Input: dimensioned drawing with shaded views. Units: mm. Origin: part minimum x, y, z. A direction names the side the tool comes from. Coordinates: 2 decimals unless noted, no trailing zeros. Loops run counter-clockwise (first coordinate to the right, second up) from the corner with the lowest first, then second, coordinate; pieces in that order, holes last.
Item 1: Section query B-B, the plane y = 17. Return the cut outline in (x, z), then the cut area to 3 significant figures.
Item 2: Reachability of the marked faces 1, 2, 3 and 4 from +Z, -Z, +X, -X, +Y, -Y: full face, straight path, thin tool, end or side. Return the list, or none.
Item 3: Pin query (flat end, axial travel): pin 1 Ø8 at (x, z) = (59.5, 18) entering from +Y; pin 2 Ø3 at (y, z) = (24, 15) entering from +X; pin 3 Ø5.5 at (y, z) = (8, 73.5) entering from -X; pin 4 Ø3 at (x, z) = (3.5, 75) entering from -Y. Return the tip coordinate at first contact, or that it passes through.
Item 4: Section query A-A, the plane x = 38.5. Return the cut outline in (y, z), then the cut area to 3 significant figures.
Item 5: Section query C-C, the plane x = 91. Return the cut outline in (y, z).
Item 6: Line query: probe 1 along Z at (x, y) = (34.5, 12); probe 2 along Z at (x, y) = (29, 21.25); probe 3 along Y at (x, z) = (63.5, 80). Output: solid intervals per line, ascending.
Item 7: Pull-direction query (X, two-part tool) for the marked faces 5, 6, 7 and 8; classes: +X half, -X half, draft (parallel to the pull), parting line (faces both ways), or undercut.
Item 8: Section query D-D, the plane z = 71. Return the cut outline in (x, y).
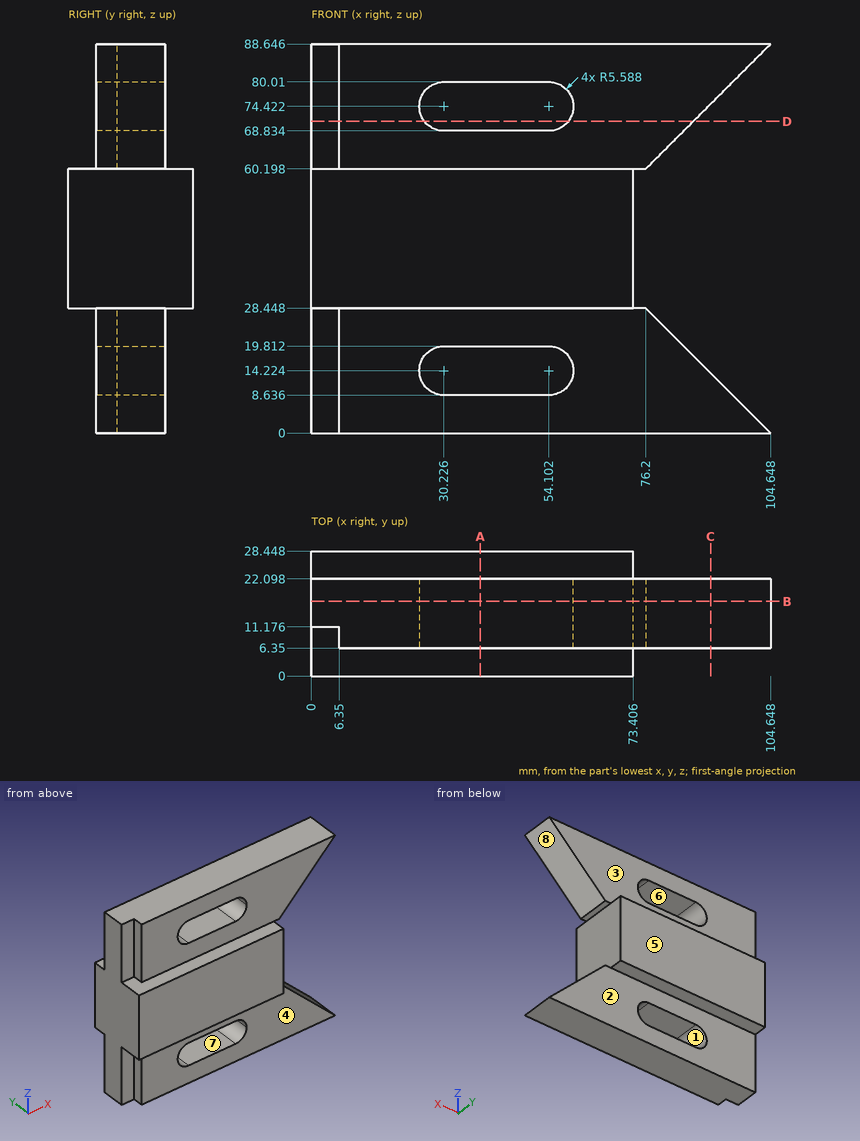
Verdict:
1. outline: (0, 0) - (104.65, 0) - (76.2, 28.45) - (73.41, 28.45) - (73.41, 60.2) - (76.2, 60.2) - (104.65, 88.65) - (0, 88.65) - close; hole (30.23, 8.64) - (54.1, 8.64) arc R5.59 ccw to (59.69, 14.22) arc R5.59 ccw to (54.1, 19.81) - (30.23, 19.81) arc R5.59 ccw to start; hole (30.23, 68.83) - (54.1, 68.83) arc R5.59 ccw to (59.69, 74.42) arc R5.59 ccw to (54.1, 80.01) - (30.23, 80.01) arc R5.59 ccw to start
1. area: 6,750 mm2
2. face 1: +Y, -Y
2. face 2: -Z, +X, -X, +Y
2. face 3: +Z, +X, -X, +Y
2. face 4: -Z, +X, -X, -Y
3. pin 1: stops at y = 22.1
3. pin 2: passes through
3. pin 3: stops at x = 6.35
3. pin 4: stops at y = 11.18
4. outline: (0, 28.45) - (6.35, 28.45) - (6.35, 19.81) - (22.1, 19.81) - (22.1, 28.45) - (28.45, 28.45) - (28.45, 60.2) - (22.1, 60.2) - (22.1, 68.83) - (6.35, 68.83) - (6.35, 60.2) - (0, 60.2) - close; (6.35, 0) - (22.1, 0) - (22.1, 8.64) - (6.35, 8.64) - close; (6.35, 80.01) - (22.1, 80.01) - (22.1, 88.65) - (6.35, 88.65) - close
4. area: 1,450 mm2
5. outline: (6.35, 0) - (22.1, 0) - (22.1, 13.65) - (6.35, 13.65) - close; (6.35, 75) - (22.1, 75) - (22.1, 88.65) - (6.35, 88.65) - close
6. probe 1: z = 0 to 8.64, 19.81 to 68.83, 80.01 to 88.65
6. probe 2: z = 0 to 8.77, 19.68 to 68.97, 79.87 to 88.65
6. probe 3: y = 6.35 to 22.1
7. face 5: draft
7. face 6: undercut
7. face 7: undercut
7. face 8: +X half
8. outline: (0, 11.18) - (6.35, 11.18) - (6.35, 6.35) - (25.81, 6.35) - (25.81, 22.1) - (0, 22.1) - close; (58.52, 6.35) - (87, 6.35) - (87, 22.1) - (58.52, 22.1) - close
